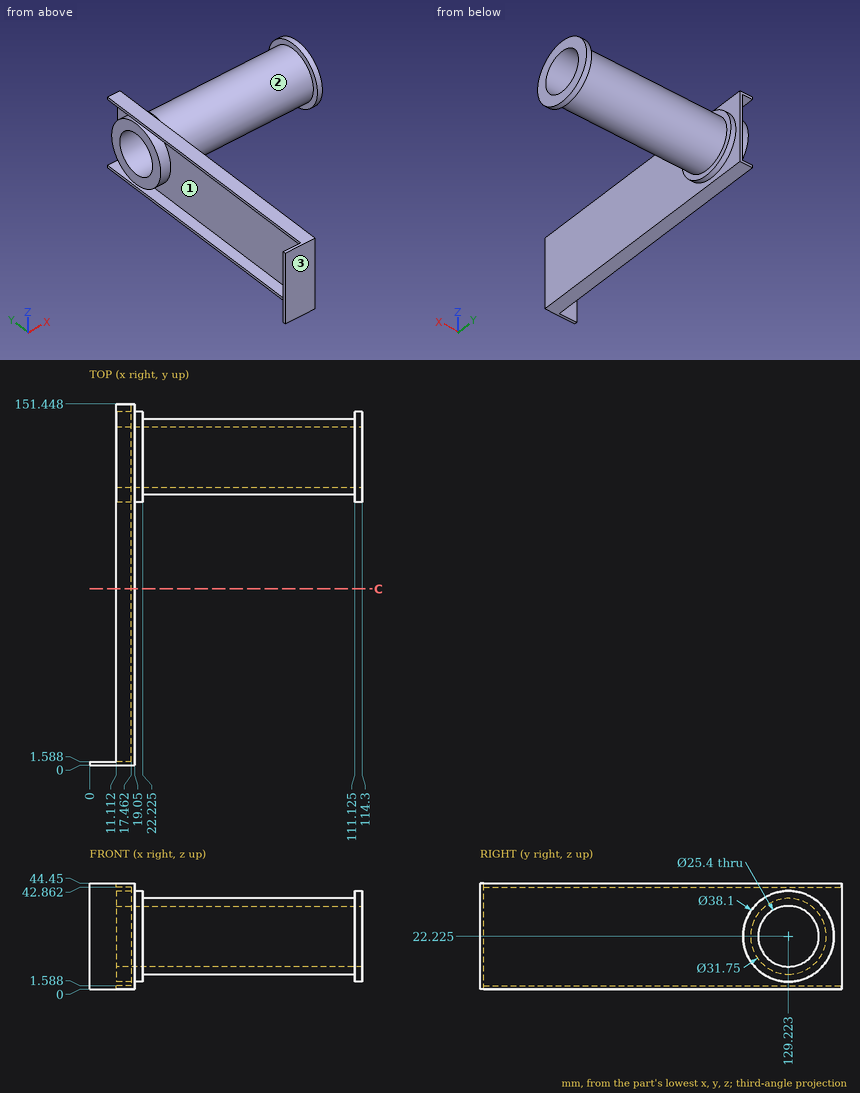
Geometry check sheet. Reference: drawing and pictorial views, mm from the part's lowest x, y, z. Round coordinates to 2 decimals unless told otherwise and drop trailing zeros. Loops run counter-clockwise (first coordinate to the right, second up) from the corner with the lowest first, then second, coordinate; pieces in that order, holes last. Notation, with made-up numbers: (41.5, -17) - (58.5, -17) arc R13 cw to (58.5, -8) - close; hole circle Ø3 at (84.25, 2.25). An arc over 180 degrees is marked (long way). Answer in a Markdown table with one row per item. Add a question column.
Q1. Gauge pin test, flat ends, axial feed: pin 1 (3 mm diameter, centred on y = 67.5, z = 27, fed in from -X); pin 2 (8 mm diameter, centred on x = 85.5, z = 25.5, fed in from -Y); pin 3 (0.5 mm diameter, centred on y = 87, z = 1, fed in from -X). Record the tip position at first contact, or that the pin passes through.
Q2. Material ranges on line 1 (Z direction, x = 14, y = 32.5); line 2 (X direction, y = 122.5, z = 39) (1 decimal); line 3 (X direction, y = 95, z = 35.5), recorded low to high.
Q3. Section check C-C on y = 74. Enter the section's corners in (x, z).
Q4. Release check for a two-part mould opening along X. For the marked faces 1, 2 and 3 record: pulls with the +X half, pulls with the -X half, needs draft (parallel to the pull), parting line crosses it, or undercut.
Found:
| question | item | result |
|---|---|---|
| 1 | pin 1 | stops at x = 17.46 |
| 1 | pin 2 | stops at y = 113.35 |
| 1 | pin 3 | stops at x = 11.11 |
| 2 | line 1 | z = 0 to 1.59, 42.86 to 44.45 |
| 2 | line 2 | x = 11.1 to 22.2, 111.1 to 114.3 |
| 2 | line 3 | x = 17.46 to 19.05 |
| 3 | outline | (11.11, 0) - (19.05, 0) - (19.05, 44.45) - (11.11, 44.45) - (11.11, 42.86) - (17.46, 42.86) - (17.46, 1.59) - (11.11, 1.59) - close |
| 4 | face 1 | pulls with the -X half |
| 4 | face 2 | undercut |
| 4 | face 3 | needs draft |
